Here's how the part is built. I have some questions about the finished solid (model axes, mm). Round coordinates to 2 decimals unless told otherwise and drop trailing zeros. Order: outer loops, then holes, each group sorted by start corner. A loop starts at its lowest first (then second) coordinate and runs counter-clockwise, first axis right, second up. Notation, with made-up numbers: (1, -24) -> (37, -24) arc R22 cw to (37, -10) -> close; hole circle Ø11 at (5, 46.5). An arc over 180 degrees is marked (long way). Answer in a Markdown table with one row per item.
```python
from build123d import *

# Parameters (mm, degrees)
SKETCH_1_W          = 150
SKETCH_1_H          = 45
EXTRUDE_1_DEPTH     = 1.5
SKETCH_2_R          = 1.6
SKETCH_2_W          = 134
SKETCH_2_H          = 13
CUT_EXTRUDE_1_DEPTH = 79.316664893
CUT_EXTRUDE_2_DEPTH = 79.316664893
FILLET_1_R          = 1.5


with BuildPart() as part:
    # 草图1 → 凸台-拉伸1 (new body)
    with BuildSketch(Plane.XY):
        Rectangle(SKETCH_1_W, SKETCH_1_H)
    extrude(amount=EXTRUDE_1_DEPTH)

    # 草图2 → 切除-拉伸1 (cut, through all)
    with BuildSketch(Plane.XY.offset(1.5)):
        with Locations((37.942286341, 17.5)):
            Circle(SKETCH_2_R)
        with Locations((57.942286341, 17.5)):
            Circle(SKETCH_2_R)
        with Locations((-37.942286341, 17.5)):
            Circle(SKETCH_2_R)
        with Locations((-57.942286341, 17.5)):
            Circle(SKETCH_2_R)
        with Locations((0, -11)):
            Rectangle(SKETCH_2_W, SKETCH_2_H)
    extrude(amount=-CUT_EXTRUDE_1_DEPTH, mode=Mode.SUBTRACT)

    # 草图3 → 切除-拉伸2 (cut, through all)
    with BuildSketch(Plane.XY.offset(1.5)):
        Polygon((-55.573181486, -0.5), (-70, 11.865844441), (-70, -0.5), align=None)
        Polygon((-38.073181486, 14.5), (-66.926818514, 14.5), (-52.5, 2.134155559), align=None)
        Polygon((-35, 11.865844441), (-49.426818514, -0.5), (-20.573181486, -0.5), align=None)
        Polygon((-3.073181486, 14.5), (-31.926818514, 14.5), (-17.5, 2.134155559), align=None)
        Polygon((0, 11.865844441), (-14.426818514, -0.5), (14.426818514, -0.5), align=None)
        Polygon((31.926818514, 14.5), (3.073181486, 14.5), (17.5, 2.134155559), align=None)
        Polygon((35, 11.865844441), (20.573181486, -0.5), (49.426818514, -0.5), align=None)
        Polygon((66.926818514, 14.5), (38.073181486, 14.5), (52.5, 2.134155559), align=None)
        Polygon((70, 11.865844441), (55.573181486, -0.5), (70, -0.5), align=None)
    extrude(amount=-CUT_EXTRUDE_2_DEPTH, mode=Mode.SUBTRACT)

    # 圆角1
    fillet_1_edges = [part.edges().sort_by_distance(p)[0] for p in [
        (17.5, 2.134155559, 0.75),
        (3.073181486, 14.5, 0.75),
        (31.926818514, 14.5, 0.75),
        (35, 11.865844441, 0.75),
        (49.426818514, -0.5, 0.75),
        (20.573181486, -0.5, 0.75),
        (-70, 11.865844441, 0.75),
        (-55.573181486, -0.5, 0.75),
        (-70, -0.5, 0.75),
        (67, -4.5, 0.75),
        (67, -17.5, 0.75),
        (-67, -17.5, 0.75),
        (-67, -4.5, 0.75),
        (-17.5, 2.134155559, 0.75),
        (-31.926818514, 14.5, 0.75),
        (-3.073181486, 14.5, 0.75),
        (75, -22.5, 0.75),
        (-75, -22.5, 0.75),
        (0, 11.865844441, 0.75),
        (14.426818514, -0.5, 0.75),
        (-75, 22.5, 0.75),
        (-14.426818514, -0.5, 0.75),
        (75, 22.5, 0.75),
        (-52.5, 2.134155559, 0.75),
        (-66.926818514, 14.5, 0.75),
        (-38.073181486, 14.5, 0.75),
        (-35, 11.865844441, 0.75),
        (-20.573181486, -0.5, 0.75),
        (-49.426818514, -0.5, 0.75),
        (52.5, 2.134155559, 0.75),
        (38.073181486, 14.5, 0.75),
        (66.926818514, 14.5, 0.75),
        (55.573181486, -0.5, 0.75),
        (70, 11.865844441, 0.75),
        (70, -0.5, 0.75),
    ]]
    fillet(fillet_1_edges, radius=FILLET_1_R)


solid = part.part
```
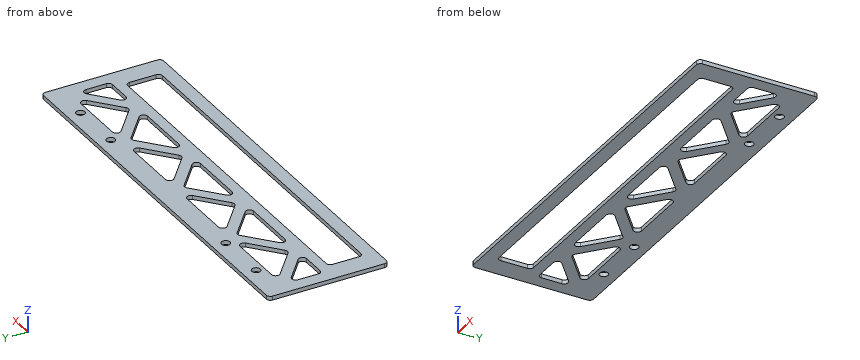
1. Suppose I cut it at D-D on z = 0.8. State how many separate pieces and enclosed holes the cut face has, then the cut area to 3 significant figures.
Numbers:
| item | result |
|---|---|
| separate pieces | 1 |
| enclosed holes | 14 |
| area | 3,610 mm2 |
2. Suppose I cut it at C-C on x = -3. Write out the boundary of the cut face in (y, z), then the cut area to 3 significant figures.
Numbers:
| item | result |
|---|---|
| outline | (-22.5, 0) -> (-17.5, 0) -> (-17.5, 1.5) -> (-22.5, 1.5) -> close; (-4.5, 0) -> (-0.5, 0) -> (-0.5, 1.5) -> (-4.5, 1.5) -> close; (9.29, 0) -> (22.5, 0) -> (22.5, 1.5) -> (9.29, 1.5) -> close |
| area | 33.3 mm2 |
3. Please list where these lines run through material, in increasing order: line 1 along Y through (x, z) = (-40.5, 0.65); line 2 along Y through (x, z) = (51.5, 1.15); line 3 along X through (y, z) = (-16, 0.15).
Numbers:
| item | result |
|---|---|
| line 1 | y = -22.5 to -17.5, -4.5 to -0.5, 7.15 to 22.5 |
| line 2 | y = -22.5 to -17.5, -4.5 to 2.99, 14.5 to 22.5 |
| line 3 | x = -75 to -67, 67 to 75 |
4. Suppose I cut it at A-A on y = -9.5. Write out the boundary of the cut face in (x, z), then the cut area to 3 significant figures.
Numbers:
| item | result |
|---|---|
| outline | (-75, 0) -> (-67, 0) -> (-67, 1.5) -> (-75, 1.5) -> close; (67, 0) -> (75, 0) -> (75, 1.5) -> (67, 1.5) -> close |
| area | 24.0 mm2 |
5. Suppose I cut it at B-B on y = 17.5. Write out the boundary of the cut face in (x, z).
Numbers:
| item | result |
|---|---|
| outline | (-75, 0) -> (-59.54, 0) -> (-59.54, 1.5) -> (-75, 1.5) -> close; (-56.34, 0) -> (-39.54, 0) -> (-39.54, 1.5) -> (-56.34, 1.5) -> close; (-36.34, 0) -> (36.34, 0) -> (36.34, 1.5) -> (-36.34, 1.5) -> close; (39.54, 0) -> (56.34, 0) -> (56.34, 1.5) -> (39.54, 1.5) -> close; (59.54, 0) -> (75, 0) -> (75, 1.5) -> (59.54, 1.5) -> close |
6. For pin 1 Ø1.9 at (x, y) = (-57.94, 17.5) entering from -Z, with a flat end and sliding along its axis, tell me the tip position at first contact or that it passes through.
Numbers:
| item | result |
|---|---|
| pin 1 | passes through |
